from build123d import *

# Parameters (mm, degrees)
F0_R     = 10.75
F0_R_2   = 8
F1_DEPTH = 25
F2_DEPTH = 2
F3_SIZE  = 0.5


with BuildPart() as f1:
    # F0 (on Top) → F1 (new body)
    with BuildSketch(Plane.XY):
        Circle(F0_R)
        Circle(F0_R_2, mode=Mode.SUBTRACT)
        Circle(F0_R_2)
    extrude(amount=F1_DEPTH)

    # F0 (on Top) → F2 (cut)
    with BuildSketch(Plane.XY):
        Circle(F0_R_2)
    extrude(amount=F2_DEPTH, mode=Mode.SUBTRACT)

    # F3
    f3_edges = [f1.edges().sort_by_distance(p)[0] for p in [
        (-10.75, 0, 25),
    ]]
    chamfer(f3_edges, length=F3_SIZE)


solid = f1.part
Read the model definition and answer for the solid it produces. Units are mm, in the model's axes. A direction names the side the tool comes from. Round coordinates to 2 decimals unless told otherwise and drop trailing zeros. Write each loop counter-clockwise with the first axis right and the second up, starting at its lowest first coordinate (ties: lowest second). Pieces come first, ordered by that corner, then holes. Notation, with made-up numbers: (67, -19.75) - (78, -19.75) arc R18 ccw to (78, -11.75) - close; hole circle Ø2 at (-13, 6.5). An arc over 180 degrees is marked (long way). Use a Markdown table: item, result.
(1) Each of these flat-tipped pins is pushed along its axis until it touches: pin 1 Ø8 at (x, y) = (-2, -0.5) entering from -Z; pin 2 Ø5 at (x, z) = (-7, 12.5) entering from -Y; pin 3 Ø2 at (x, z) = (3, 13.5) entering from -Y. Where does it stop, or does it pass through?
Reported:
| item | result |
|---|---|
| pin 1 | z = 2 |
| pin 2 | y = -9.76 |
| pin 3 | y = -10.56 |
(2) The part is cut by section A-A (x = 0). Write down the section's boundary in (y, z).
Reported:
| item | result |
|---|---|
| outline | (-10.75, 0) - (-8, 0) - (-8, 2) - (8, 2) - (8, 0) - (10.75, 0) - (10.75, 24.5) - (10.25, 25) - (-10.25, 25) - (-10.75, 24.5) - close |
(3) The part is cut by section C-C (z = 3). Write down the section's boundary in (x, y).
Reported:
| item | result |
|---|---|
| outline | circle Ø21.5 at (0, 0) |
(4) The mould has two halves that part along Y. Classify faces 3 (the flat face through (0, 0, 2)), 4 (the flat face through (-2, 8, 0)), 5 (the cylindrical face through (-1.4, 10.66, 12.08)): released by +Y, released by -Y, zero draft, split by the parting line, or undercut.
Reported:
| item | result |
|---|---|
| face 3 | undercut |
| face 4 | zero draft |
| face 5 | split by the parting line |
(5) Straight lines are drawn through the part: line 1 along Y through (x, z) = (0, 1.2); line 2 along Z through (x, y) = (-3.25, -5.75); line 3 along X through (y, z) = (-3.25, 7.5). For each, find the intervals that lie inside material, in ascending order. Write a range as [from, to].
Reported:
| item | result |
|---|---|
| line 1 | [-10.75, -8], [8, 10.75] |
| line 2 | [2, 25] |
| line 3 | [-10.25, 10.25] |
(6) Which of the six approach directions +Z, -Z, +X, -X, +Y, -Y give full straight-line access (tool end or side, diameter ignored) to faces 1 (the cylindrical face through (-1.73, -7.81, 0.99)), 2 (the flat face through (0, 0, 25))?
Reported:
| item | result |
|---|---|
| face 1 | -Z |
| face 2 | +Z, +X, -X, +Y, -Y |
